Build history of the part. All positions in model axes, mm. A direction names the side the tool comes from. Give positions to 0.01 mm unless a question says otherwise; leave off trailing zeros. Loops run counter-clockwise (first coordinate to the right, second up) from the corner with the lowest first, then second, coordinate; pieces in that order, holes last. Notation, with made-up numbers: (1.5, 70) -> (26.5, 70) arc R21 ccw to (26.5, 91) -> close; hole circle Ø2 at (-34, -40). An arc over 180 degrees is marked (long way). Answer as a JSON object with one key per item and string values. Group by question number.
from build123d import *

# Parameters (mm, degrees)
CUT_EXTRUDE1_DEPTH = 5
SKETCH5_R          = 1
CUT_EXTRUDE3_DEPTH = 25.777841371


with BuildPart() as part:
    # Sketch1 → Revolve1 (revolve)
    with BuildSketch(Plane.XY, mode=Mode.PRIVATE) as revolve1_sk:
        Polygon((3.175, 0), (3.175, 12), (11.5, 12), (10, 10.5), (10, 3), (11.5, 3), (11.5, 0), align=None)
    revolve(revolve1_sk.sketch.rotate(Axis((0, 0, 0), (0, 1, 0)), 90), axis=Axis((0, 0, 0), (0, 1, 0)))

    # Sketch2 → Cut-Extrude1 (cut)
    with BuildSketch(Plane(origin=(0, 12, 0), x_dir=(1, 0, 0), z_dir=(0, 1, 0))):
        Polygon((3.207902433, 5.55625), (-3.207902433, 5.55625), (-6.415804866, 0), (-3.207902433, -5.55625), (3.207902433, -5.55625), (6.415804866, 0), align=None)
    extrude(amount=-CUT_EXTRUDE1_DEPTH, mode=Mode.SUBTRACT)

    # Sketch5 → Cut-Extrude3 (cut, through all)
    with BuildSketch(Plane(origin=(4.81185365, 0, 2.778125), x_dir=(-0.5000000000000006, 0, 0.8660254037844384), z_dir=(-0.8660254037844384, 0, -0.5000000000000006))):
        with Locations((0, 8)):
            Circle(SKETCH5_R)
    extrude(amount=-CUT_EXTRUDE3_DEPTH, mode=Mode.SUBTRACT)


solid = part.part
(1) Saw through at B-B on y = 5.75. List the corners of the cut face in (x, z) (3 decimals), plus the area to 3 significant figures.
(2) Saw through at A-A on x = 0. List the corners of the cut face in (y, z) (3 decimals), plus the area to 3 significant figures.
(3) Probe line 1 along X through (y, z) = (2.75, 0) (3 decimals); line 2 along X through (y, z) = (3.5, 0) (3 decimals); line 3 along Y through (x, z) = (8.5, 6). List the from-to ranges inside material, lowest first. Write a range as [from, to].
(4) Saw through at C-C on y = 7.5. List the corners of the cut face in (x, z), plus the area to 3 significant figures.
(5) Pin check, flat tips, straight feed: pin 1 (1.5 mm diameter, centred on x = 1, y = 10, fed in from -Z); pin 2 (5 mm diameter, centred on x = -5, y = 8.5, fed in from +Z); pin 3 (6 mm diameter, centred on x = 2, z = 1.5, fed in from +Y). Stop position of each tip, or through.
(6) 3-axis set-ups, long thin cutter, end or side, ignore diameter. For faces 1 (the flat face through (0, 10, 5.556)), 2 (the cylindrical face through (0, 7, 10)), 3 (the cylindrical face through (1.93, 3.55, 2.52)): which of +Z, -Z, +X, -X, +Y, -Y reach the whole face in a straight line?
(7) Pull direction Y, two halves, no side cores. Call faces 4 (the flat face through (-5, 3, -9)), 5 (the cylindrical face through (7, 9, 4)), 6 (the flat face through (4.8, 9.5, 2.8)), 7 (the flat face through (2.4, 0, -2.4)): pulls with the +Y half, pulls with the -Y half, needs draft (parallel to the pull), parting line crosses it, or undercut.
Calculated:
{
 "1": {"outline": "circle Ø20 at (0, 0); hole circle Ø6.35 at (0, 0)", "area": "282 mm^2"},
 "2": {"outline": "(0, -11.5) -> (3, -11.5) -> (3, -10) -> (10.5, -10) -> (12, -11.5) -> (12, -5.556) -> (7, -5.556) -> (7, -3.175) -> (0, -3.175) -> close; (0, 3.175) -> (7, 3.175) -> (7, 5.556) -> (12, 5.556) -> (12, 11.5) -> (10.5, 10) -> (3, 10) -> (3, 11.5) -> (0, 11.5) -> close", "area": "151 mm^2"},
 "3": {"line 1": "x = [-11.5, -3.175], [3.175, 11.5]", "line 2": "x = [-10, -3.175], [3.175, 10]", "line 3": "y = [0, 3], [10.9, 12]"},
 "4": {"outline": "(-6.42, 0) -> (-3.21, 5.56) -> (3.21, 5.56) -> (4.38, 3.53) -> (8.19, 5.73) arc R10 ccw (long way) to (9.06, 4.23) -> (5.24, 2.03) -> (6.42, 0) -> (3.21, -5.56) -> (-3.21, -5.56) -> close", "area": "200 mm^2"},
 "5": {"pin 1": "stops at z = -10.2", "pin 2": "stops at z = 9.68", "pin 3": "stops at y = 7"},
 "6": {"face 1": "+Y", "face 2": "none", "face 3": "+Y, -Y"},
 "7": {"face 4": "undercut", "face 5": "undercut", "face 6": "needs draft", "face 7": "pulls with the -Y half"}
}
